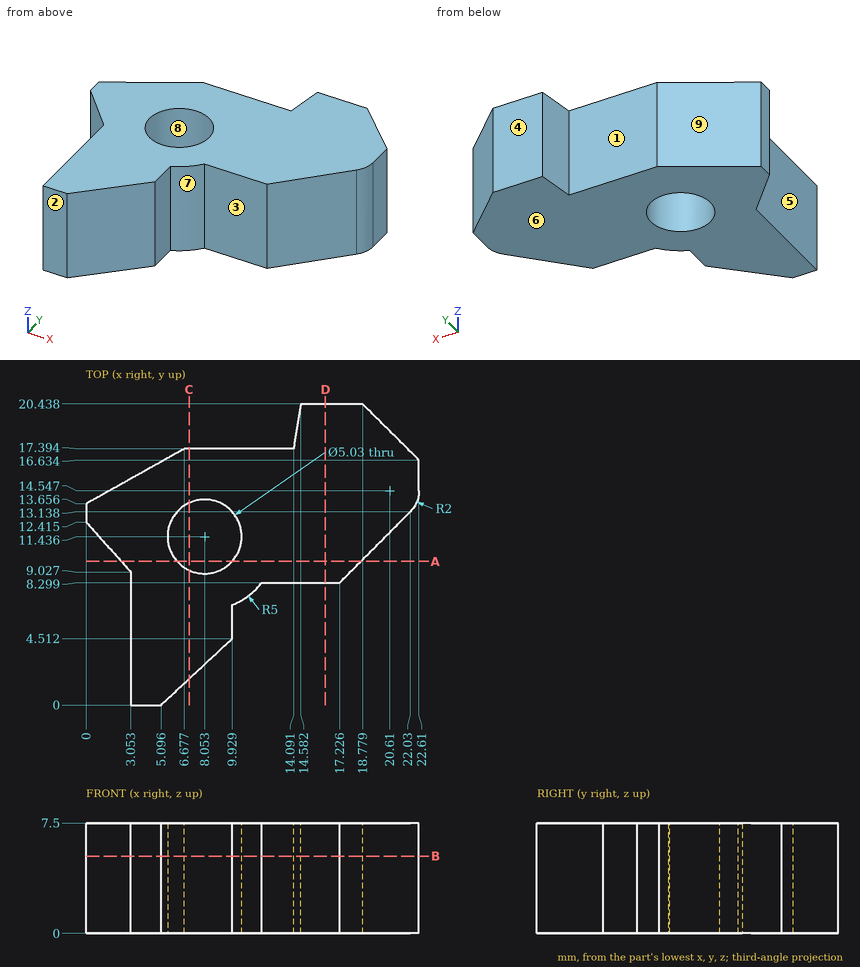
Geometry: see drawing. Coordinates: mm, zero at the bounding-box minimum. A direction names the side the tool comes from. Give positions to 0.01 mm unless a question says otherwise; leave off trailing zeros. Loops run counter-clockwise (first coordinate to the right, second up) from the corner with the lowest first, then second, coordinate; pieces in that order, holes last. Notation, with made-up numbers: M 28,-14.75 L 69,-14.75 A20 ccw 69,10.25 Z; hole C 10,-27 d4. An arc over 180 degrees is marked long. Use one line per item in the form item = value.
1. Line query: L1, parallel to Y at x = 14, z = 6; L2, parallel to X at y = 5, z = 3.25; L3, parallel to X at y = 12, z = 6.5 (1 decimal). Output: solid intervals per line, ascending.
Numbers:
L1 = 8.3 to 17.39
L2 = 3.05 to 9.93
L3 = 0.4 to 5.6, 10.5 to 20.9
2. Section query D-D, the plane x = 16.25. Return the cut outline in (y, z).
Numbers:
outline = M 8.3,0 L 20.44,0 L 20.44,7.5 L 8.3,7.5 Z
3. Section query B-B, the plane z = 5.25. Return the cut outline in (x, y) (1 decimal).
Numbers:
outline = M 0,12.4 L 3.1,9 L 3.1,0 L 5.1,0 L 9.9,4.5 L 9.9,6.8 A5 ccw 11.9,8.3 L 17.2,8.3 L 22,13.1 A2 ccw 22.6,14.5 L 22.6,16.6 L 18.8,20.4 L 14.6,20.4 L 14.1,17.4 L 6.7,17.4 L 0,13.7 Z; hole C 8.1,11.4 d5
4. Section query A-A, the plane y = 9.75. Return the cut outline in (x, z).
Numbers:
outline = M 2.4,0 L 6.19,0 L 6.19,7.5 L 2.4,7.5 Z; M 9.92,0 L 18.67,0 L 18.67,7.5 L 9.92,7.5 Z
5. Section query C-C, the plane x = 7. Return the cut outline in (y, z).
Numbers:
outline = M 1.78,0 L 9.15,0 L 9.15,7.5 L 1.78,7.5 Z; M 13.72,0 L 17.39,0 L 17.39,7.5 L 13.72,7.5 Z
6. First-contact query: pin 1 (6 mm diameter, centred on x = 8.05, y = 11.44, fed in from +Z); pin 2 (3 mm diameter, centred on y = 10.5, z = 5.5, fed in from -X) (1 decimal); pin 3 (4 mm diameter, centred on x = 15, z = 4, fed in from -Y); pin 4 (4 mm diameter, centred on x = 6, z = 2, fed in from +Y). Flat tips, straight axial feed; report the tip coordinate or a pass-through.
Numbers:
pin_1 = 7.5
pin_2 = 0.4
pin_3 = 8.3
pin_4 = 17.39
7. Pull-direction query (Y, two-part tool) for the marked faces 6, 7, 8 and 9; classes: released by +Y, released by -Y, zero draft, split by the parting line, or undercut.
Numbers:
face_6 = zero draft
face_7 = released by -Y
face_8 = undercut
face_9 = released by +Y
8. Reachability of the marked faces 1, 2, 3, 4 and 5 from +Z, -Z, +X, -X, +Y, -Y: full face, straight path, thin tool, end or side. Return the list, or none.
Numbers:
face_1 = +Z, -Z, -X, +Y
face_2 = +Z, -Z, +X, -X, -Y
face_3 = +Z, -Z, +X, -Y
face_4 = +Z, -Z, +X, -X, +Y
face_5 = +Z, -Z, -X, -Y
